```python
from build123d import *

# Parameters (mm, degrees)
SKETCH2_W       = 8.4
SKETCH2_H       = 1.5
SLOT_DEPTH      = 1.3
THDSCHPAT_COUNT = 15
THDSCHPAT_PITCH = 0.685714286


with BuildPart() as part:
    # BodySke → Base-Revolve (revolve)
    with BuildSketch(Plane.XY, mode=Mode.PRIVATE) as base_revolve_sk:
        Polygon((0, 0), (0, 4.2), (0.5, 4.2), (2.7, 2), (13, 2), (13, 0), align=None)
    revolve(base_revolve_sk.sketch.rotate(Axis((-6.35, 0, 0), (1, 0, 0)), 90), axis=Axis((-6.35, 0, 0), (1, 0, 0)))

    # Sketch2 → Slot (cut)
    with BuildSketch(Plane.ZY):
        Rectangle(SKETCH2_W, SKETCH2_H)
    extrude(amount=-SLOT_DEPTH, mode=Mode.SUBTRACT)

    # ThdSchSke → ThreadSchematic (revolve, cut)
    with BuildSketch(Plane.XY):
        Polygon((3.400001, -1.61), (3.12692006, -2), (3.12692006, -2.5), (3.67308194, -2.5), (3.67308194, -2), align=None)
    threadschematic = revolve(axis=Axis((-3.175, 0, 0), (1, 0, 0)), mode=Mode.SUBTRACT)

    # ThdSchPat: ThreadSchematic ×15
    with Locations(*[(i * THDSCHPAT_PITCH, 0, 0) for i in range(1, THDSCHPAT_COUNT)]):
        add(threadschematic, mode=Mode.SUBTRACT)


solid = part.part
```
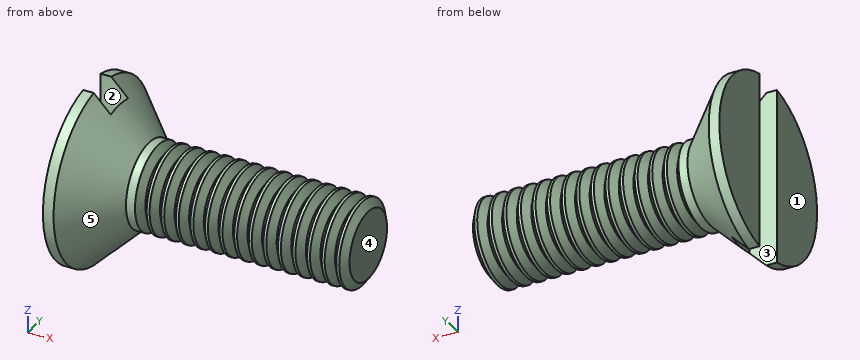
The listing builds one solid part. Answer for the finished solid, in the listing's coordinates (mm). Face numbers are marked on the shaded views. A direction names the side the tool comes from. Give positions to 0.01 mm unless a question says otherwise; leave off trailing zeros. Answer in a Markdown table with one row per item. Add a question column.
Q1. For a pull along Y with two mould halves and no side action, classify the marked faces 3, 4 and 5 as released by +Y, released by -Y, zero draft, split by the parting line, or undercut.
Q2. Find the intervals of material crossed by line 1 along X through (y, z) = (0.5, -1.25); line 2 along Z through (x, y) = (1.5, -1.25); line 3 along Y through (x, z) = (12, -1.5), in increasing order. Write a range as [from, to].
Q3. Which of the six approach directions +Z, -Z, +X, -X, +Y, -Y give full straight-line access (tool end or side, diameter ignored) to the marked faces 1 and 2?
Q4. Given P1, Ø3, axis at x = 7, y = 3, coming from the +Z side; P2, Ø4, axis at x = 8.5, z = 1.5, coming from the +Y side; P3, Ø4, axis at x = 11.5, z = -3, coming from the -Y side, each flat-ended and moving along its own axis, determine where each tip first touches the part or whether it passes through.
Determined:
| question | item | result |
|---|---|---|
| 1 | face 3 | undercut |
| 1 | face 4 | zero draft |
| 1 | face 5 | split by the parting line |
| 2 | line 1 | x = [1.3, 13] |
| 2 | line 2 | z = [-2.95, 2.95] |
| 2 | line 3 | y = [-1.32, 1.32] |
| 3 | face 1 | +Z, -Z, -X, +Y, -Y |
| 3 | face 2 | +Z, -Z, -X |
| 4 | P1 | stops at z = 1.32 |
| 4 | P2 | stops at y = 2 |
| 4 | P3 | stops at y = -1.73 |
